Work out the finished part from the listing and answer in its coordinate system (mm). A direction names the side the tool comes from. Round coordinates to 2 decimals unless told otherwise and drop trailing zeros. Loops run counter-clockwise (first coordinate to the right, second up) from the corner with the lowest first, then second, coordinate; pieces in that order, holes last. Notation, with made-up numbers: (67, -30.5) -> (88, -30.5) arc R23 cw to (88, -11.5) -> close; hole circle Ø4 at (-32, 27). An arc over 180 degrees is marked (long way). Use CSV: the item, a comma, the result in double quotes. Start each with the question number.
from build123d import *

# Parameters (mm, degrees)
F1_DEPTH = 63.5
F0_W     = 25.347986334
F0_H     = 19.05
F2_DEPTH = 25.4
F3_DEPTH = 7.9375
F5_R     = 6.35


with BuildPart() as f1:
    # F0 (on Front) → F1 (new body, symmetric)
    with BuildSketch(Plane.XZ):
        Polygon((-41.275, 9.525), (-41.275, -9.525), (41.275, -9.525), (41.275, 9.525), (22.225, 9.525), align=None)
    extrude(amount=F1_DEPTH, both=True)

    # F0 (on Front) → F2 (join, symmetric)
    with BuildSketch(Plane.XZ):
        with BuildLine():
            Line((22.225, 9.525), (41.275, 9.525))
            Line((41.275, 9.525), (41.275, 27.0002))
            ThreePointArc((41.275, 27.0002), (45.9246798487, 38.2255201513), (57.15, 42.8752))
            Line((57.15, 42.8752), (60.325, 42.8752))
            Line((60.325, 42.8752), (60.325, 61.9252))
            Line((60.325, 61.9252), (57.15, 61.9252))
            add(Edge.make_bspline(
                [(56.4854564208, 61.9188770487), (56.7077656128, 61.9217360058), (56.9292858392, 61.9238445309), (57.15, 61.9252)],
                knots=[110.8436997421, 110.8436997421, 110.8436997421, 110.8436997421, 111.5045361635, 111.5045361635, 111.5045361635, 111.5045361635], degree=3))
            ThreePointArc((56.4854564208, 61.9188770487), (32.2204511723, 51.4598242868), (22.225, 27.0002))
            Line((22.225, 27.0002), (22.225, 9.525))
        make_face()
        with Locations((72.998993167, 52.4002)):
            Rectangle(F0_W, F0_H)
    extrude(amount=F2_DEPTH, both=True)

    # F0 (on Front) → F3 (join, symmetric)
    with BuildSketch(Plane.XZ):
        with BuildLine():
            add(Edge.make_bspline(
                [(-41.275, 9.525), (-40.2883552222, 39.8470173814), (19.1969951279, 61.4393372205), (56.4854564208, 61.9188770487)],
                knots=[0, 0, 0, 0, 110.8436997421, 110.8436997421, 110.8436997421, 110.8436997421], degree=3))
            Line((-41.275, 9.525), (22.225, 9.525))
            Line((22.225, 9.525), (22.225, 27.0002))
            ThreePointArc((22.225, 27.0002), (32.2204511723, 51.4598242868), (56.4854564208, 61.9188770487))
        make_face()
    extrude(amount=F3_DEPTH, both=True)

    # F0 (on Front) → F4 (revolve)
    with BuildSketch(Plane.XZ):
        Polygon((111.125, 66.675), (85.6816321611, 66.675), (85.725, 38.1), (111.125, 38.1), align=None)
    revolve(axis=Axis((85.7033160806, 0, 52.3875), (-0.0015176829, 0, 0.9999988483)))

    # F5
    f5_edges = [f1.edges().sort_by_distance(p)[0] for p in [
        (41.275, -63.5, 0),
        (-41.275, -63.5, 0),
        (41.275, 63.5, 0),
        (-41.275, 63.5, 0),
    ]]
    fillet(f5_edges, radius=F5_R)


solid = f1.part
Q1. Straight lines are drawn through the part: line 1 (Z direction, x = 73.5, y = 25); line 2 (Z direction, x = 32.5, y = 34) (3 decimals); line 3 (X direction, y = 9, z = 22.5) (3 decimals). For each, find the intervals that lie inside material, in ascending order. Write a range as from..to.
Q2. Each of these flat-tipped pins is pushed along its axis until it touches: pin 1 (10 mm diameter, centred on x = 77, z = 52, fed in from +Y); pin 2 (5 mm diameter, centred on y = -5, z = 27, fed in from +X); pin 3 (8.5 mm diameter, centred on y = -14, z = 21.5, fed in from -X) (3 decimals). Where does it stop, or does it pass through?
Q3. Section B-B, the plane y = -37 is taken. Write down the section's boundary in (x, z) (3 decimals), and give its area (3 significant figures).
Q4. Which of the six approach directions +Z, -Z, +X, -X, +Y, -Y give full straight-line access (tool end or side, diameter ignored) to faces 1 (the conical face through (109.2, -9.7, 52.6)), 2 (the flat face through (-3, -7.938, 30)), 3 (the cylindrical face through (32.49, 16.55, 51.73)), 4 (the cylindrical face through (45.8, -0.4, 38.1))?
Q5. Section A-A, the plane z = 0 is taken. Write down the section's boundary in (x, y) (3 decimals).
Report:
1,line 1,"z = 42.88..61.93"
1,line 2,"z = -9.525..9.525"
1,line 3,"x = 22.225..41.275"
2,pin 1,"stops at y = 25.4"
2,pin 2,"stops at x = 41.47"
2,pin 3,"stops at x = 22.225"
3,outline,"(-41.275, -9.525) -> (41.275, -9.525) -> (41.275, 9.525) -> (-41.275, 9.525) -> close"
3,area,"1,570 mm²"
4,face 1,"none"
4,face 2,"+Z, -X, -Y"
4,face 3,"+Z, -X, +Y"
4,face 4,"-Z, +Y, -Y"
5,outline,"(-41.275, -57.15) arc R6.35 ccw to (-34.925, -63.5) -> (34.925, -63.5) arc R6.35 ccw to (41.275, -57.15) -> (41.275, 57.15) arc R6.35 ccw to (34.925, 63.5) -> (-34.925, 63.5) arc R6.35 ccw to (-41.275, 57.15) -> close"
